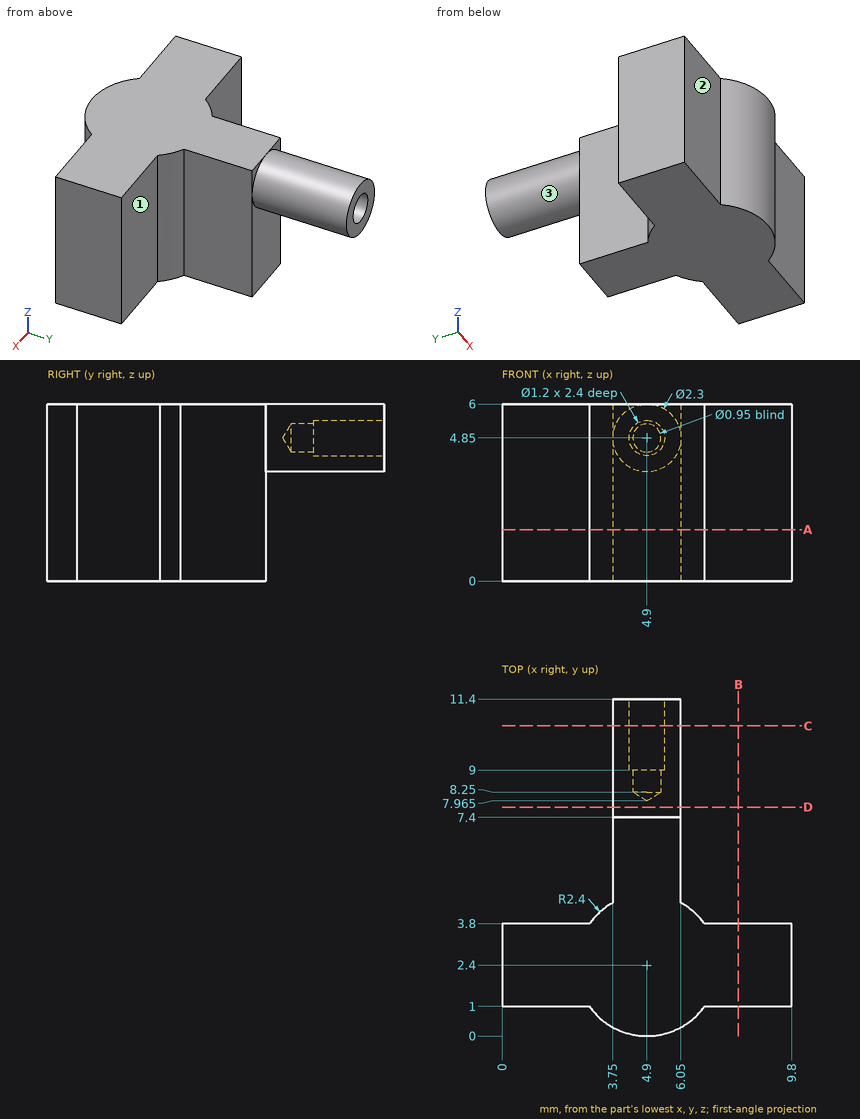
Design review of the part shown in the three views and the two pictorial views. Dimensions are in mm from the part's minimum x, y and z. A direction names the side the tool comes from. Coordinates: 2 decimals unless noted, no trailing zeros. Order: outer loops, then holes, each group sorted by start corner. A loop starts at its lowest first (then second) coordinate and runs counter-clockwise, first axis right, second up. Notation, with made-up numbers: (18.25, -7) - (37.25, -7) arc R22 ccw to (37.25, 4) - close; hole circle Ø5 at (-30, 43). An arc over 180 degrees is marked (long way). One line per question, with ' | ' between items.
Q1. Clearance check with flat-ended pins moving along their axes: pin 1 Ø2.5 at (x, z) = (8, 4) entering from +Y; pin 2 Ø1 at (x, y) = (1.5, 6.5) entering from -Z; pin 3 Ø1.5 at (x, z) = (2, 3) entering from -Y; pin 4 Ø2.5 at (y, z) = (6, 3.5) entering from +X. State where each tip first meets the part, or that it passes through.
Answer key:
pin 1: stops at y = 3.93 | pin 2: passes through | pin 3: stops at y = 1 | pin 4: stops at x = 6.05
Q2. To check wall thickness, follow line 1 along X through (y, z) = (10.3, 4.85); line 2 along Y through (x, z) = (1.5, 5.5); line 3 along X through (y, z) = (6.75, 4.5). State the ranges of each line that lie inside material, in increasing order.
Answer key:
line 1: x = 3.75 to 4.3, 5.5 to 6.05 | line 2: y = 1 to 3.8 | line 3: x = 3.75 to 6.05
Q3. For the marked faces 1, 2 and 3, list the 3-axis set-ups (+Z, -Z, +X, -X, +Y, -Y) from which the entire face can be reached by the end or side of a thin tool; tool diameter is ignored.
Answer key:
face 1: +Z, -Z, +X, +Y | face 2: +Z, -Z, -X, -Y | face 3: +Y
Q4. Consider section C-C, the plane y = 10.5. Give the boundary of the cut face in (x, z).
Answer key:
outline: circle Ø2.3 at (4.9, 4.85); hole circle Ø1.2 at (4.9, 4.85)
Q5. Consider section A-A, the plane z = 1.75. Give the boundary of the cut face in (x, y), then the cut area to 3 significant figures.
Answer key:
outline: (0, 1) - (2.95, 1) arc R2.4 ccw to (6.85, 1) - (9.8, 1) - (9.8, 3.8) - (6.85, 3.8) arc R2.4 ccw to (6.05, 4.51) - (6.05, 7.4) - (3.75, 7.4) - (3.75, 4.51) arc R2.4 ccw to (2.95, 3.8) - (0, 3.8) - close | area: 39.1 mm2
Q6. Consider section D-D, the plane y = 7.75. Give the boundary of the cut face in (x, z).
Answer key:
outline: circle Ø2.3 at (4.9, 4.85)
Q7. Consider section B-B, the plane x = 8. Give the boundary of the cut face in (y, z).
Answer key:
outline: (1, 0) - (3.8, 0) - (3.8, 6) - (1, 6) - close
